```python
from build123d import *

# Parameters (mm, degrees)
SKETCH_1_W          = 400
SKETCH_1_H          = 260
EXTRUDE_1_DEPTH     = 5
CUT_EXTRUDE_1_DEPTH = 239.589605809
SKETCH_3_R          = 1.55
SKETCH_3_R_2        = 10
SKETCH_3_R_3        = 3
CUT_EXTRUDE_2_DEPTH = 239.589605809


with BuildPart() as part:
    # 草圖1 → 填料-伸長1 (new body)
    with BuildSketch(Plane(origin=(0, 0, 0), x_dir=(1, 0, 0), z_dir=(0, 1, 0))):
        Rectangle(SKETCH_1_W, SKETCH_1_H)
    extrude(amount=EXTRUDE_1_DEPTH)

    # 草圖2 → 除料-伸長1 (cut, through all)
    with BuildSketch(Plane(origin=(0, 5, 0), x_dir=(1, 0, 0), z_dir=(0, 1, 0))):
        with BuildLine():
            Line((-182.75, 115), (-182.75, -115))
            ThreePointArc((-182.75, -115), (-185, -117.25), (-187.25, -115))
            Line((-187.25, -115), (-187.25, 115))
            ThreePointArc((-187.25, 115), (-185, 117.25), (-182.75, 115))
        make_face()
        with BuildLine():
            Line((182.75, 115), (182.75, -115))
            ThreePointArc((182.75, -115), (185, -117.25), (187.25, -115))
            Line((187.25, -115), (187.25, 115))
            ThreePointArc((187.25, 115), (185, 117.25), (182.75, 115))
        make_face()
    extrude(amount=-CUT_EXTRUDE_1_DEPTH, mode=Mode.SUBTRACT)

    # 草圖3 → 除料-伸長2 (cut, through all)
    with BuildSketch(Plane(origin=(0, 5, 0), x_dir=(1, 0, 0), z_dir=(0, 1, 0))):
        with Locations(Location((-15.5, 85.5, 0), (0, 0, 270))):
            Circle(SKETCH_3_R)
        with Locations(Location((15.5, 85.5, 0), (0, 0, 270))):
            Circle(SKETCH_3_R)
        with Locations(Location((-15.5, 54.5, 0), (0, 0, 270))):
            Circle(SKETCH_3_R)
        with Locations(Location((15.5, 54.5, 0), (0, 0, 270))):
            Circle(SKETCH_3_R)
        with Locations(Location((0, 70, 0), (0, 0, 270))):
            Circle(SKETCH_3_R_2)
        with Locations(Location((-124.304765272, 70, 0), (0, 0, 270))):
            Circle(SKETCH_3_R_3)
        with Locations(Location((124.304765272, 70, 0), (0, 0, 90))):
            Circle(SKETCH_3_R_3)
        with Locations(Location((0, -54.304765272, 0), (0, 0, 270))):
            Circle(SKETCH_3_R_3)
    extrude(amount=-CUT_EXTRUDE_2_DEPTH, mode=Mode.SUBTRACT)


solid = part.part
```
Can you work these out from the model? Positions are in its coordinate system, mm. Give positions to 0.01 mm unless a question says otherwise; leave off trailing zeros. Write each loop counter-clockwise with the first axis right and the second up, starting at its lowest first coordinate (ties: lowest second). Pieces come first, ordered by that corner, then holes. Notation, with made-up numbers: (81, 4) - (127, 4) arc R28 ccw to (127, 38) - close; hole circle Ø10 at (44, -20). An arc over 180 degrees is marked (long way). Write item = value, one per line. Start each with the question number.
1. For pin 1 (5.5 mm diameter, centred on x = -124.3, z = -70, fed in from -Y) (3 decimals), with a flat end and sliding along its axis, tell me the tip position at first contact or that it passes through.
2. Please list where these lines run through material, in increasing order: line 1 (X direction, y = 3.55, z = -85.5); line 2 (X direction, y = 0.35, z = -94.5); line 3 (X direction, y = 2.75, z = -70).
3. Imagine slicing it at A-A (z = -15.5). Please give me the cut outline in (x, y), and give its area (4 significant figures).
4. Imagine slicing it at B-B (y = 3.6). Count the separate pieces of the cut face and the enclosed holes in it, and give its area (3 significant figures).
Worked answers:
q1.pin_1 = through
q2.line_1 = -200 to -187.25, -182.75 to -17.05, -13.95 to 13.95, 17.05 to 182.75, 187.25 to 200
q2.line_2 = -200 to -187.25, -182.75 to 182.75, 187.25 to 200
q2.line_3 = -200 to -187.25, -182.75 to -127.3, -121.3 to -10, 10 to 121.3, 127.3 to 182.75, 187.25 to 200
q3.outline = (-200, 0) - (-187.25, 0) - (-187.25, 5) - (-200, 5) - close; (-182.75, 0) - (182.75, 0) - (182.75, 5) - (-182.75, 5) - close; (187.25, 0) - (200, 0) - (200, 5) - (187.25, 5) - close
q3.area = 1,955 mm2
q4.separate_pieces = 1
q4.enclosed_holes = 10
q4.area = 101,000 mm2
